Design review of the part built by this model. Coordinates are the model's own, in mm. A direction names the side the tool comes from. Round coordinates to 2 decimals unless told otherwise and drop trailing zeros. Write each loop counter-clockwise with the first axis right and the second up, starting at its lowest first coordinate (ties: lowest second). Pieces come first, ordered by that corner, then holes. Notation, with made-up numbers: M -28.75,36.25 L -13.75,36.25 A33 ccw -13.75,73.25 Z; hole C 47.5,66 d1. An arc over 180 degrees is marked long. One line per question, with ' | ' between items. Start each with the question number.
Item 1: Insertion check: pin 1 Ø2.5 at (x, z) = (-110, -1.5) entering from -Y; pin 2 Ø1.5 at (x, z) = (-103.5, -77.5) entering from -Y; pin 3 Ø12 at (y, z) = (0.5, -45.5) entering from -X; pin 4 Ø4 at (x, y) = (-102.5, 5) entering from +Z. Each pin has a flat end and moves straight along its axis. Give the tip position at first contact, or say it passes through.
Item 2: Draft analysis for pull direction Y (two halves, no side actions). For faces 1 (the face through (-113.634, 55.468, -2.535)), 2 (the face through (-102, 19.721, -76)), 3 (the face through (-112, 51, -5)), 4 (the face through (-101.347, 69.402, -39.287)), state which applies: released by +Y, released by -Y, zero draft, split by the parting line, or undercut.
Item 3: Machinability: for faces 5 (the face through (-112, 41.4, -3)), 6 (the face through (-112, -61.958, -3)), 7 (the face through (-102, -1, -72.689)), which of the approach directions +Z, -Z, +X, -X, +Y, -Y give a long, thin tool a straight path to every point of the face, cutting with its end or side? Answer none if there is none.
Item 4: Add section C-C, the plane z = -49.5. State the section outline as (x, y) points, and give its area (3 significant figures).
Item 5: Add section D-D, the plane y = 8. State the section outline as (x, z) points.
Item 6: Add section B-B, the plane x = -102.5. State the section outline as (y, z) points.
Item 7: For L1, parallel to Y at x = -106, z = -4.5; L2, parallel to Z at x = -106, y = 43.5; L3, parallel to X at y = -4, z = -18, list the stretches that pass through material, from the lowest coordinate up.
Item 8: Add section A-A, the plane y = 44. State the section outline as (x, z) points, and give its area (3 significant figures).
```python
from build123d import *

# Parameters (mm, degrees)
CROQUIS2_W              = 200
CROQUIS2_H              = 150
CROQUIS2_R              = 2
CROQUIS2_R_2            = 2.5
CROQUIS2_W_2            = 31.297292299
CROQUIS2_H_2            = 43.768728426
CROQUIS2_H_3            = 43.768728427
CROQUIS2_W_3            = 23.573907934
CROQUIS2_H_4            = 45.323962431
SALIENTE_EXTRUIR1_DEPTH = 2
REDONDEO1_R             = 10
BOSS_EXTRUDE1_DEPTH     = 25
SKETCH3_W               = 62.040442094
SKETCH3_H               = 5.530821024
BOSS_EXTRUDE2_DEPTH     = 22
SKETCH8_W               = 62.040442094
SKETCH8_H               = 5.530821024
BOSS_EXTRUDE6_DEPTH     = 13
SKETCH2_W               = 200
SKETCH2_H               = 78.124132015
SKETCH2_W_2             = 62.040442094
SKETCH2_H_2             = 5.530821024
BOSS_EXTRUDE3_DEPTH     = 5
SKETCH4_W               = 62.040442094
SKETCH4_H               = 5.530821024
BOSS_EXTRUDE4_DEPTH     = 19
SKETCH5_W               = 7.442573222
SKETCH5_H               = 2.991451355
BOSS_EXTRUDE5_DEPTH     = 21
SKETCH6_R               = 2.5
CUT_EXTRUDE1_DEPTH      = 158.961544101
FILLET1_R               = 10
SKETCH10_W              = 79.68896036
SKETCH10_H              = 143.358595358
BOSS_EXTRUDE7_DEPTH     = 5
SKETCH11_W              = 5
SKETCH11_H              = 20
BOSS_EXTRUDE13_DEPTH    = 14
SKETCH12_R              = 2.5
CUT_EXTRUDE2_DEPTH      = 176.118897221
FILLET2_R               = 6
CUT_EXTRUDE3_DEPTH      = 222.270727407
SKETCH14_W              = 12
SKETCH14_H              = 2
CUT_EXTRUDE4_DEPTH      = 198.082327879
SKETCH15_W              = 7
SKETCH15_H              = 40
CUT_EXTRUDE5_DEPTH      = 10


with BuildPart() as part:
    # Croquis2 → Saliente-Extruir1 (new body)
    with BuildSketch(Plane.XY):
        with Locations((0.108263467, -0.36008145)):
            Rectangle(CROQUIS2_W, CROQUIS2_H)
        with Locations((89.108263467, -66.5)):
            Circle(CROQUIS2_R, mode=Mode.SUBTRACT)
        with Locations((-88.891736533, -66.5)):
            Circle(CROQUIS2_R, mode=Mode.SUBTRACT)
        with Locations(Location((89.108263467, 65.779837101, 0), (0, 0, 180))):
            Circle(CROQUIS2_R, mode=Mode.SUBTRACT)
        with Locations(Location((-88.891736533, 65.779837101, 0), (0, 0, 180))):
            Circle(CROQUIS2_R, mode=Mode.SUBTRACT)
        with Locations((-80.865436179, -59.36008145)):
            Circle(CROQUIS2_R_2, mode=Mode.SUBTRACT)
        with Locations((81.108263467, -59.36008145)):
            Circle(CROQUIS2_R_2, mode=Mode.SUBTRACT)
        with Locations(Location((81.108263467, 58.63991855, 0), (0, 0, 180))):
            Circle(CROQUIS2_R_2, mode=Mode.SUBTRACT)
        with Locations(Location((-80.865436179, 58.63991855, 0), (0, 0, 180))):
            Circle(CROQUIS2_R_2, mode=Mode.SUBTRACT)
        with BuildLine():
            Line((-62.091736533, 70.63991855), (64.108263467, 70.63991855))
            ThreePointArc((64.108263467, 70.63991855), (66.108263467, 68.63991855), (64.108263467, 66.63991855))
            Line((64.108263467, 66.63991855), (-62.091736533, 66.63991855))
            ThreePointArc((-62.091736533, 66.63991855), (-64.091736533, 68.63991855), (-62.091736533, 70.63991855))
        make_face(mode=Mode.SUBTRACT)
        Polygon((-71.391736533, -12.902447307), (-71.391736533, 12.182284408), (-79.241736533, 12.28991855), (-83.891736533, 12.28991855), (-83.891736533, -13.01008145), (-79.241736533, -13.01008145), align=None, mode=Mode.SUBTRACT)
        with BuildLine():
            Line((92.108263467, 45.478381757), (92.108263467, -46.198544657))
            ThreePointArc((92.108263467, -46.198544657), (90.807295546, -47.897576736), (89.108263467, -46.596608814))
            Line((89.108263467, -46.596608814), (89.108263467, 45.876445915))
            ThreePointArc((89.108263467, 45.876445915), (90.807295546, 47.177413836), (92.108263467, 45.478381757))
        make_face(mode=Mode.SUBTRACT)
        Polygon((84.108263467, 12.28991855), (84.108263467, -13.01008145), (79.458263467, -13.01008145), (71.608263467, -13.01008145), (71.608263467, 12.28991855), (79.458263467, 12.28991855), align=None, mode=Mode.SUBTRACT)
        with BuildLine():
            Line((-91.891736533, 45.478381757), (-91.891736533, -46.198544657))
            ThreePointArc((-91.891736533, -46.198544657), (-90.590768612, -47.897576736), (-88.891736533, -46.596608814))
            Line((-88.891736533, -46.596608814), (-88.891736533, 45.876445915))
            ThreePointArc((-88.891736533, 45.876445915), (-90.590768612, 47.177413836), (-91.891736533, 45.478381757))
        make_face(mode=Mode.SUBTRACT)
        with Locations((-30.011405388, 36.299005811)):
            Rectangle(CROQUIS2_W_2, CROQUIS2_H_2, mode=Mode.SUBTRACT)
        with BuildLine():
            Line((-62.091736533, -71.36008145), (64.108263467, -71.36008145))
            ThreePointArc((64.108263467, -71.36008145), (66.108263467, -69.36008145), (64.108263467, -67.36008145))
            Line((64.108263467, -67.36008145), (-62.091736533, -67.36008145))
            ThreePointArc((-62.091736533, -67.36008145), (-64.091736533, -69.36008145), (-62.091736533, -71.36008145))
        make_face(mode=Mode.SUBTRACT)
        with Locations((-30.011405388, -26.799059535)):
            Rectangle(CROQUIS2_W_2, CROQUIS2_H_3, mode=Mode.SUBTRACT)
        with Locations((12.982877294, -0.693345879)):
            Rectangle(CROQUIS2_W_3, CROQUIS2_H_4, mode=Mode.SUBTRACT)
    extrude(amount=SALIENTE_EXTRUIR1_DEPTH)

    # Redondeo1
    redondeo1_edges = [part.edges().sort_by_distance(p)[0] for p in [
        (100.108263467, -75.36008145, 1),
        (-99.891736533, -75.36008145, 1),
        (-99.891736533, 74.63991855, 1),
        (100.108263467, 74.63991855, 1),
    ]]
    fillet(redondeo1_edges, radius=REDONDEO1_R)

    # Sketch1 → Boss-Extrude1 (add)
    with BuildSketch(Plane.XY.offset(2)):
        Polygon((-67.071845217, 64.63991855), (-67.071845217, 60.63991855), (-8.841198185, 60.63991855), (-8.841198185, 3.63991855), (-67.071845217, 3.63991855), (-67.071845217, -0.36008145), (-8.841198185, -0.36008145), (-8.841198185, -53.36008145), (-67.071845217, -53.36008145), (-67.071845217, -57.574734434), (-5.031403123, -57.574734434), (-5.031403123, -40.931443482), (46.608263467, -40.931443482), (46.608263467, -36.931443482), (-5.031403123, -36.931443482), (-5.031403123, 30.068556518), (46.608263467, 30.068556518), (46.608263467, 34.068556518), (-5.031403123, 34.068556518), (-5.031403123, 64.63991855), align=None)
    extrude(amount=BOSS_EXTRUDE1_DEPTH)

    # Sketch3 → Boss-Extrude2 (add)
    with BuildSketch(Plane.XZ.offset(57.574734434)):
        with Locations((-36.05162417, 24.234589488)):
            Rectangle(SKETCH3_W, SKETCH3_H)
    extrude(amount=BOSS_EXTRUDE2_DEPTH)

    # Sketch8 → Boss-Extrude6 (add)
    with BuildSketch(Plane(origin=(0, 64.63991855, 0), x_dir=(1, 0, 0), z_dir=(0, 1, 0))):
        with Locations((-36.05162417, -24.234589488)):
            Rectangle(SKETCH8_W, SKETCH8_H)
    extrude(amount=BOSS_EXTRUDE6_DEPTH)

    # Sketch2 → Boss-Extrude3 (add)
    with BuildSketch(Plane.XZ.offset(75.36008145)):
        with Locations((0.108263467, 41.062066008)):
            Rectangle(SKETCH2_W, SKETCH2_H)
        with Locations((-36.05162417, 24.234589488)):
            Rectangle(SKETCH2_W_2, SKETCH2_H_2, mode=Mode.SUBTRACT)
    extrude(amount=-BOSS_EXTRUDE3_DEPTH)

    # Sketch4 → Boss-Extrude4 (add)
    with BuildSketch(Plane(origin=(0, 64.63991855, 0), x_dir=(1, 0, 0), z_dir=(0, 1, 0))):
        with Locations((-36.05162417, -24.234589488)):
            Rectangle(SKETCH4_W, SKETCH4_H)
    extrude(amount=BOSS_EXTRUDE4_DEPTH)

    # Sketch5 → Boss-Extrude5 (add)
    with BuildSketch(Plane.XZ.offset(75.36008145)):
        with Locations((-80.540187187, 3.495725678)):
            Rectangle(SKETCH5_W, SKETCH5_H)
        with Locations((80.756714122, 3.495725678)):
            Rectangle(SKETCH5_W, SKETCH5_H)
    extrude(amount=BOSS_EXTRUDE5_DEPTH)

    # Sketch6 → Cut-Extrude1 (cut, through all)
    with BuildSketch(Plane.XY.offset(4.991451355)):
        with Locations((-80.996023003, -59.284349751)):
            Circle(SKETCH6_R)
        with Locations((81.166025964, -59.051385225)):
            Circle(SKETCH6_R)
    extrude(amount=-CUT_EXTRUDE1_DEPTH, mode=Mode.SUBTRACT)

    # Fillet1
    # the kernel refuses this fillet: 10 mm, written as the material it takes off along each edge
    with BuildSketch(Plane(origin=(100.108263467, -70.36008145, 2), x_dir=(-1, 0, 0), z_dir=(0, 0, 1)), Plane(origin=(-99.891736533, -70.36008145, 101.77476711), x_dir=(1, 0, 0), z_dir=(0, 0, -1))) as fillet1_piece_1:
        with BuildLine():
            CenterArc((8.660254038, 10), FILLET1_R, 210, 60)
            Line((0, 5), (0, 0))
            Line((0, 0), (8.660254038, 0))
        make_face()
    extrude(amount=99.77476711, mode=Mode.SUBTRACT)


with BuildPart() as body_2:
    # Sketch10 → Boss-Extrude7 (new body)
    with BuildSketch(Plane.ZY.offset(99.891736533)):
        with Locations((-39.84448018, -0.278985798)):
            Rectangle(SKETCH10_W, SKETCH10_H)
    extrude(amount=BOSS_EXTRUDE7_DEPTH)

    # Sketch11 → Boss-Extrude13 (add)
    with BuildSketch(Plane.ZY.offset(104.891736533)):
        with Locations((-2.5, -51.958283477)):
            Rectangle(SKETCH11_W, SKETCH11_H)
        with Locations((-2.5, 51.400311881)):
            Rectangle(SKETCH11_W, SKETCH11_H)
    extrude(amount=BOSS_EXTRUDE13_DEPTH)


with BuildPart() as cut_extrude2_tool:
    # Sketch12 → Cut-Extrude2 (new, through all)
    with BuildSketch(Plane(origin=(0, 0, -5), x_dir=(-1, 0, 0), z_dir=(0, 0, -1))):
        with Locations((94.306850379, -54.336044589)):
            Circle(SKETCH12_R)
        with Locations((94.306850379, 53.778072993)):
            Circle(SKETCH12_R)
        with Locations((115.476622686, 53.778072993)):
            Circle(SKETCH12_R)
        with Locations((113.140977594, -49.445291065)):
            Circle(SKETCH12_R)
    extrude(amount=-CUT_EXTRUDE2_DEPTH)


with BuildPart() as part_1:
    add(part.part)

    # Cut-Extrude2: cut by cut_extrude2_tool
    add(cut_extrude2_tool.part, mode=Mode.SUBTRACT)

    # Sketch13 → Cut-Extrude3 (cut, through all)
    with BuildSketch(Plane.XY.offset(80.124132015)):
        Polygon((-88.891736533, 41.400311881), (-87.891736533, 41.400311881), (-87.891736533, 63.52554782), (-99.891736533, 63.52554782), (-99.891736533, 94.010082764), (108.48763668, 94.010082764), (108.48763668, -102.123784964), (-99.891736533, -102.123784964), (-99.891736533, -61.922986139), (-88.478309969, -61.922986139), (-88.478309969, -40.956005085), (-99.891736533, -40.956005085), (-99.891736533, 41.400311881), align=None)
    extrude(amount=-CUT_EXTRUDE3_DEPTH, mode=Mode.SUBTRACT)


with BuildPart() as body_2_1:
    add(body_2.part)

    # Cut-Extrude2: cut by cut_extrude2_tool
    add(cut_extrude2_tool.part, mode=Mode.SUBTRACT)

    # Fillet2
    # the kernel refuses this fillet: 6 mm, written as the material it takes off along each edge
    with BuildSketch(Plane(origin=(-99.891736533, -71.958283477, -94.479159818), x_dir=(0, 1, 0), z_dir=(0, 0, 1))) as fillet2_piece_1:
        with BuildLine():
            CenterArc((5.916079783, 6), FILLET2_R, 189.594068227, 80.405931773)
            Line((0, 5), (-0.118321596, 4.98))
            ThreePointArc((-0.118321596, 4.98), (-0.12, 2.5), (-0.12, 0))
            Line((-0.12, 0), (0, -0.12))
            Line((0, -0.12), (5.916079783, -0.12))
            Line((5.916079783, -0.12), (5.916079783, 0))
        make_face()
    extrude(amount=109.269359275, mode=Mode.SUBTRACT)
    with BuildSketch(Plane(origin=(-99.891736533, 71.400311881, 14.790199458), x_dir=(-1, 0, 0), z_dir=(0, 0, -1))) as fillet2_piece_2:
        with BuildLine():
            CenterArc((6, -5.916079783), FILLET2_R, 99.594068227, 80.405931773)
            Line((0, -5.916079783), (-0.12, -5.916079783))
            Line((-0.12, -5.916079783), (-0.12, 0))
            Line((-0.12, 0), (0, 0.12))
            ThreePointArc((0, 0.12), (2.5, 0.12), (4.98, 0.118321596))
            Line((4.98, 0.118321596), (5, 0))
        make_face()
    extrude(amount=109.269359275, mode=Mode.SUBTRACT)

    # Sketch15 → Cut-Extrude5 (cut)
    with BuildSketch(Plane.ZY.offset(104.891736533)):
        with Locations((-76.18896036, -0.278985798)):
            Rectangle(SKETCH15_W, SKETCH15_H)
    extrude(amount=-CUT_EXTRUDE5_DEPTH, mode=Mode.SUBTRACT)


with BuildPart() as cut_extrude3_piece_1:
    # of the separate pieces the step leaves, piece 1, a body of its own (cut_extrude3_pieces)
    add(part_1.part.solids().sort_by_distance((-99.891736533, 63.52554782, 0))[0])


with BuildPart() as cut_extrude3_piece_2:
    # of the separate pieces the step leaves, piece 2, a body of its own (cut_extrude3_pieces)
    add(part_1.part.solids().sort_by_distance((-99.891736533, -40.956005085, 0))[0])


with BuildPart() as cut_extrude4_tool:
    # Sketch14 → Cut-Extrude4 (new, through all)
    with BuildSketch(Plane(origin=(0, 63.52554782, 0), x_dir=(1, 0, 0), z_dir=(0, 1, 0))):
        with Locations((-93.891736533, -1)):
            Rectangle(SKETCH14_W, SKETCH14_H)
    extrude(amount=-CUT_EXTRUDE4_DEPTH)


with BuildPart() as cut_extrude3_piece_1_1:
    add(cut_extrude3_piece_1.part)

    # Cut-Extrude4: cut by cut_extrude4_tool
    add(cut_extrude4_tool.part, mode=Mode.SUBTRACT)


with BuildPart() as cut_extrude3_piece_2_1:
    add(cut_extrude3_piece_2.part)

    # Cut-Extrude4: cut by cut_extrude4_tool
    add(cut_extrude4_tool.part, mode=Mode.SUBTRACT)


solid = body_2_1.part
```
Computed values:
1) pin 1: stops at y = -61.96 | pin 2: stops at y = -71.81 | pin 3: stops at x = -104.89 | pin 4: stops at z = 0
2) face 1: undercut | face 2: undercut | face 3: zero draft | face 4: released by +Y
3) face 5: +Z, -Z, -X | face 6: +Z, -Z, -X, -Y | face 7: -Z, +X, -X
4) outline: M -104.89,-71.96 A6 ccw -99.89,-66.04 L -99.89,65.48 A6 ccw -104.89,71.4 Z | area: 702 mm^2
5) outline: M -104.89,-72.69 L -99.89,-72.69 L -99.89,0 L -104.89,0 Z
6) outline: M -70.99,-79.69 L -20.28,-79.69 L -20.28,-72.69 L 19.72,-72.69 L 19.72,-79.69 L 70.43,-79.69 L 70.43,0 L -70.99,0 Z
7) L1: y = -61.96 to -41.96, 41.4 to 61.4 | L2: z = -5 to 0 | L3: x = -104.89 to -99.89
8) outline: M -118.89,-5 L -104.89,-5 L -104.89,-79.69 L -99.89,-79.69 L -99.89,0 L -118.89,0 Z | area: 468 mm^2
